Design review of the part built by this model. Coordinates are the model's own, in mm. A direction names the side the tool comes from. Round coordinates to 2 decimals unless told otherwise and drop trailing zeros. Order: outer loops, then holes, each group sorted by start corner. A loop starts at its lowest first (then second) coordinate and runs counter-clockwise, first axis right, second up.
from build123d import *

# Parameters (mm, degrees)
SKETCH1_W           = 32.5
SKETCH1_H           = 7.5
BOSS_EXTRUDE1_DEPTH = 2
SKETCH2_R           = 7
SKETCH2_R_2         = 5
BOSS_EXTRUDE2_DEPTH = 7.5
SKETCH3_R           = 1
CUT_EXTRUDE1_DEPTH  = 3.18
FILLET1_R           = 2


with BuildPart() as part:
    # Sketch1 → Boss-Extrude1 (new body)
    with BuildSketch(Plane.XY):
        Rectangle(SKETCH1_W, SKETCH1_H)
    extrude(amount=BOSS_EXTRUDE1_DEPTH)

    # Sketch2 → Boss-Extrude2 (add)
    with BuildSketch(Plane(origin=(0, 3.75, 0), x_dir=(1, 0, 0), z_dir=(0, 1, 0))):
        with Locations((0, 6)):
            Circle(SKETCH2_R)
        with Locations(Location((0, 6, 0), (0, 0, 180))):
            Circle(SKETCH2_R_2, mode=Mode.SUBTRACT)
    extrude(amount=-BOSS_EXTRUDE2_DEPTH)

    # Sketch3 → Cut-Extrude1 (cut)
    with BuildSketch(Plane(origin=(0, 0, 0), x_dir=(-1, 0, 0), z_dir=(0, 0, -1))):
        with Locations((-12.28, 0)):
            Circle(SKETCH3_R)
        with Locations((12.28, 0)):
            Circle(SKETCH3_R)
    extrude(amount=-CUT_EXTRUDE1_DEPTH, mode=Mode.SUBTRACT)

    # Fillet1
    fillet1_edges = [part.edges().sort_by_distance(p)[0] for p in [
        (-16.25, 3.75, 1),
        (16.25, 3.75, 1),
        (16.25, -3.75, 1),
        (-16.25, -3.75, 1),
    ]]
    fillet(fillet1_edges, radius=FILLET1_R)


solid = part.part
1) Take a section at C-C on x = 0. Give the boundary of the cut face in (y, z).
Results:
outline: (-3.75, -13) - (3.75, -13) - (3.75, -11) - (-3.75, -11) - close; (-3.75, -1) - (3.75, -1) - (3.75, 2) - (-3.75, 2) - close
2) Take a section at D-D on x = -10. Give the boundary of the cut face in (y, z), plus the area to 3 significant figures.
Results:
outline: (-3.75, 0) - (3.75, 0) - (3.75, 2) - (-3.75, 2) - close
area: 15.0 mm2
3) To check wall thickness, follow line 1 along Y through (x, z) = (12.28, 0.9); line 2 along X through (y, z) = (-0.5, 0.5); line 3 along Z through (x, y) = (8, -1.25). State the ranges of each line that lie inside material, in increasing order.
Results:
line 1: y = -3.75 to -1, 1 to 3.75
line 2: x = -16.25 to -13.15, -11.41 to 11.41, 13.15 to 16.25
line 3: z = 0 to 2
4) Take a section at B-B on z = -6. Give the boundary of the cut face in (x, y), plus the area to 3 significant figures.
Results:
outline: (-7, -3.75) - (-5, -3.75) - (-5, 3.75) - (-7, 3.75) - close; (5, -3.75) - (7, -3.75) - (7, 3.75) - (5, 3.75) - close
area: 30.0 mm2
5) Take a section at A-A on y = 0. Give the boundary of the cut face in (x, z), plus the area to 3 significant figures.
Results:
outline: (-16.25, 0) - (-13.28, 0) - (-13.28, 2) - (-16.25, 2) - close; (-11.28, 0) - (-3.61, 0) arc R7 ccw (long way) to (3.61, 0) - (11.28, 0) - (11.28, 2) - (-11.28, 2) - close; (13.28, 0) - (16.25, 0) - (16.25, 2) - (13.28, 2) - close; hole circle Ø10 at (0, -6)
area: 128 mm2
6) For faces 1 (the face through (-10, 0, 0)), 2 (the face through (10, 0, 0)), 3 (the face through (4, 0, -9)), list the 3-axis set-ups (+Z, -Z, +X, -X, +Y, -Y) from which the entire face can be reached by the end or side of a thin tool; tool diameter is ignored.
Results:
face 1: -X, +Y, -Y
face 2: +X, +Y, -Y
face 3: +Y, -Y
7) The part is to be moulded in two halves that separate along Y. For faces 4 (the face through (-16.25, 0, 1)), 5 (the face through (15.65, 3.18, 1.01)), 6 (the face through (-11.28, 0.04, 0.99)), say which applies: released by +Y, released by -Y, zero draft, split by the parting line, or undercut.
Results:
face 4: zero draft
face 5: released by +Y
face 6: undercut
